Answer from the drawing. Dimensions are ordinates in mm from the lowest x, y and z of the part. Coordinates: 2 decimals unless noted, no trailing zeros. Order: outer loops, then holes, each group sorted by start corner. A loop starts at its lowest first (then second) coordinate and runs counter-clockwise, first axis right, second up. Notation, with made-up numbers: (43.5, -32) -> (48.5, -32) arc R9 cw to (48.5, -24) -> close; hole circle Ø3 at (-26.75, 9.5). An arc over 180 degrees is marked (long way). Answer as a JSON object with one key per item and string values. Group by question number.
1) Section B-B on z = 1 is taken. Count the separate pieces of the cut face and the enclosed holes in it, and give its area (3 significant figures).
2) Section C-C on x = 30 is taken. Determine the outline of the cut face in (y, z) (1 decimal).
3) Consider L1, parallel to Y at x = 24, z = 0.7 (1 decimal); L2, parallel to X at y = 55.5, z = 0.4 (1 decimal); L3, parallel to Y at x = 14, z = 0.9 (1 decimal). Determine where each line is inside the solid, lowest interval first.
4) Section A-A on y = 33 is taken. Determine the outline of the cut face in (x, z).
5) Given pin 1 (3 mm diameter, centred on x = 42.04, y = 16.65, fed in from -Z), flat-ended and moving along its own axis, determine where the tip first touches the part or whether it passes through.
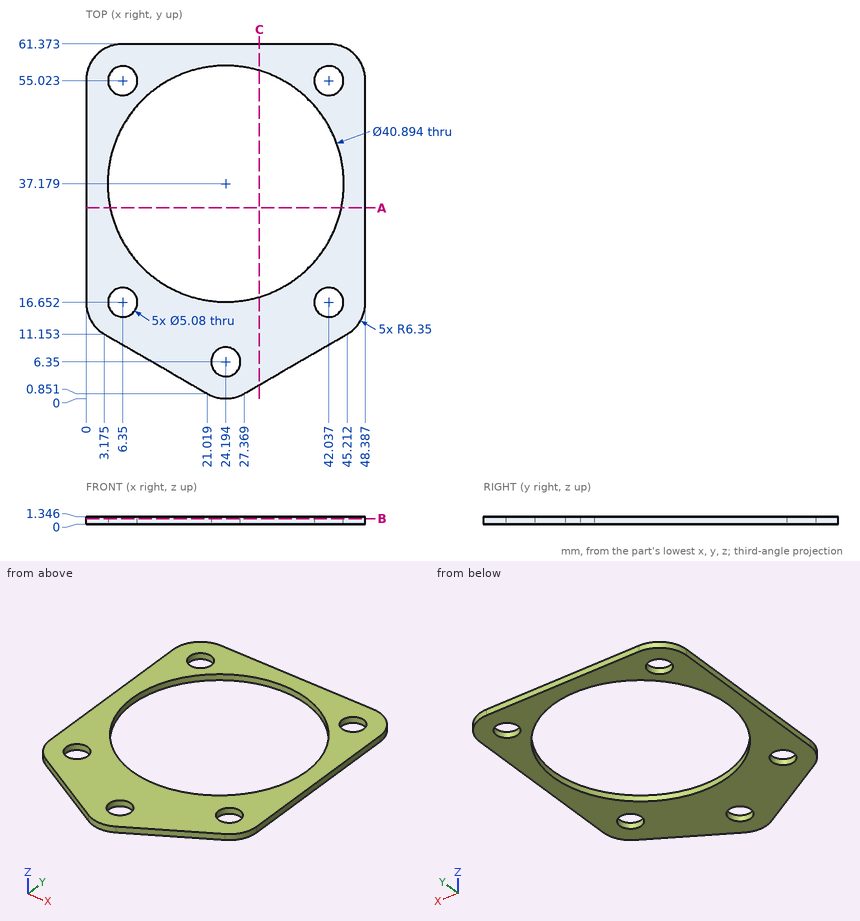
Worked answers:
{
 "1": {"separate pieces": "1", "enclosed holes": "6", "area": "1,240 mm²"},
 "2": {"outline": "(2.4, 0) -> (17.6, 0) -> (17.6, 1.3) -> (2.4, 1.3) -> close; (56.8, 0) -> (61.4, 0) -> (61.4, 1.3) -> (56.8, 1.3) -> close"},
 "3": {"L1": "y = 0 to 3.8, 8.9 to 16.7, 57.6 to 61.4", "L2": "x = 0 to 3.9, 8.8 to 15.1, 33.3 to 39.5, 44.5 to 48.4", "L3": "y = 4.9 to 19.5, 54.9 to 61.4"},
 "4": {"outline": "(0, 0) -> (4.18, 0) -> (4.18, 1.35) -> (0, 1.35) -> close; (44.21, 0) -> (48.39, 0) -> (48.39, 1.35) -> (44.21, 1.35) -> close"},
 "5": {"pin 1": "passes through"}
}
